Here's how the part is built. I have some questions about the finished solid (model axes, mm). A direction names the side the tool comes from. Give positions to 0.01 mm unless a question says otherwise; leave off trailing zeros. Write each loop counter-clockwise with the first axis right and the second up, starting at its lowest first coordinate (ties: lowest second). Pieces come first, ordered by that corner, then holes. Notation, with made-up numbers: (1, 41.25) - (17, 41.25) arc R24 ccw to (17, 57.25) - close; hole circle Ø3 at (44, 19). An arc over 180 degrees is marked (long way). Write each question's results on one line, items separated by ' | '. Start each with the question number.
Item 1: Please list where these lines run through material, in increasing order: line 1 along Z through (x, y) = (-62, 10); line 2 along Z through (x, y) = (-61.5, 6); line 3 along X through (y, z) = (14.5, 8.5).
Item 2: We'd pull the mould along Z, two halves only. Please class faces 4 (the cylindrical face through (0.77, 17.1, 29.14)), 5 (the cylindrical face through (0.77, 0.9, -29.14)), 6 (the cylindrical face through (-67.325, 12.466, 5.77)), 7 (the flat face through (85, 9, 3)): +Z half, -Z half, draft (parallel to the pull), parting line (faces both ways), or undercut.
Item 3: Which directions (+Z, -Z, +X, -X, +Y, -Y) give clear straight access to the entire face, cutting with the end or side of a thin tool? Please do faces 1 (the cylindrical face through (-82.46, 6.78, -3.85)), 2 (the flat face through (-85, 9, -5)), 3 (the cylindrical face through (82.465, 10.946, -12.765)).
Item 4: Will these pins go through, and if not, where does the flat tip stop? P1, Ø6, axis at x = 64.5, z = -18, coming from the +Y side; P2, Ø2, axis at y = 6.5, z = -20, coming from the -X side; P3, Ø5, axis at y = 5.5, z = 23.5, coming from the +X side.
Item 5: Suppose I cut it at A-A on x = -70. List the corners of the cut face in (y, z) for me, then the cut area to 3 significant figures.
Item 6: Suppose I cut it at B-B on z = -5. List the corners of the cut face in (x, y) for me, then the cut area to 3 significant figures.
Item 7: Suppose I cut it at C-C on z = -24. List the corners of the cut face in (x, y) for me.
```python
from build123d import *

# Parameters (mm, degrees)
SKETCH1_W           = 110
SKETCH1_H           = 60
BOSS_EXTRUDE1_DEPTH = 18
FILLET1_R           = 3
SKETCH2_R           = 3.55
BOSS_EXTRUDE2_DEPTH = 25
SKETCH3_R           = 3.55
BOSS_EXTRUDE3_DEPTH = 25
SKETCH4_R           = 2.5
BOSS_EXTRUDE4_DEPTH = 5
SKETCH5_R           = 2.5
BOSS_EXTRUDE5_DEPTH = 5


with BuildPart() as part:
    # Sketch1 → Boss-Extrude1 (new body)
    with BuildSketch(Plane(origin=(0, 0, 0), x_dir=(1, 0, 0), z_dir=(0, 1, 0))):
        Rectangle(SKETCH1_W, SKETCH1_H)
    extrude(amount=BOSS_EXTRUDE1_DEPTH)

    # Fillet1
    fillet1_edges = [part.edges().sort_by_distance(p)[0] for p in [
        (0, 18, 30),
        (0, 0, 30),
        (0, 0, -30),
        (0, 18, -30),
    ]]
    fillet(fillet1_edges, radius=FILLET1_R)

    # Sketch2 → Boss-Extrude2 (add)
    with BuildSketch(Plane(origin=(55, 0, 0), x_dir=(0, 0, -1), z_dir=(1, 0, 0))):
        with Locations(Location((13.090661553, 8.467313241, 0), (0, 0, 180))):
            Circle(SKETCH2_R)
        with Locations(Location((-3.345586855, 8.467313241, 0), (0, 0, 180))):
            Circle(SKETCH2_R)
    extrude(amount=BOSS_EXTRUDE2_DEPTH)

    # Sketch3 → Boss-Extrude3 (add)
    with BuildSketch(Plane.ZY.offset(55)):
        with Locations(Location((-15, 9, 0), (0, 0, 180))):
            Circle(SKETCH3_R)
        with Locations(Location((5, 9, 0), (0, 0, 180))):
            Circle(SKETCH3_R)
        with Locations(Location((-5, 9, 0), (0, 0, 180))):
            Circle(SKETCH3_R)
    extrude(amount=BOSS_EXTRUDE3_DEPTH)

    # Sketch4 → Boss-Extrude4 (add)
    with BuildSketch(Plane.ZY.offset(80)):
        with Locations((-15, 9)):
            Circle(SKETCH4_R)
        with Locations((-5, 9)):
            Circle(SKETCH4_R)
        with Locations((5, 9)):
            Circle(SKETCH4_R)
    extrude(amount=BOSS_EXTRUDE4_DEPTH)

    # Sketch5 → Boss-Extrude5 (add)
    with BuildSketch(Plane(origin=(80, 0, 0), x_dir=(0, 0, -1), z_dir=(1, 0, 0))):
        with Locations((-3.345586855, 8.467313241)):
            Circle(SKETCH5_R)
        with Locations((13.090661553, 8.467313241)):
            Circle(SKETCH5_R)
    extrude(amount=BOSS_EXTRUDE5_DEPTH)


solid = part.part
```
Checked values:
1) line 1: z = -18.41 to -11.59, -8.41 to -1.59, 1.59 to 8.41 | line 2: z = -16.9 to -13.1, -6.9 to -3.1, 3.1 to 6.9 | line 3: x = -55 to 55
2) face 4: +Z half | face 5: -Z half | face 6: undercut | face 7: draft
3) face 1: -X | face 2: +Z, -Z, -X, +Y, -Y | face 3: +X
4) P1: stops at y = 11.46 | P2: stops at x = -55 | P3: stops at x = 55
5) outline: circle Ø7.1 at (9, -15); circle Ø7.1 at (9, -5); circle Ø7.1 at (9, 5) | area: 119 mm^2
6) outline: (-85, 6.5) - (-80, 6.5) - (-80, 5.45) - (-55, 5.45) - (-55, 0) - (55, 0) - (55, 18) - (-55, 18) - (-55, 12.55) - (-80, 12.55) - (-80, 11.5) - (-85, 11.5) - close | area: 2,180 mm^2
7) outline: (-55, 0) - (55, 0) - (55, 18) - (-55, 18) - close
